For this review, take the finished solid that the model builds, in its own axes (mm). A direction names the side the tool comes from. Round coordinates to 2 decimals unless told otherwise and drop trailing zeros. Write each loop counter-clockwise with the first axis right and the second up, starting at its lowest first coordinate (ties: lowest second). Pieces come first, ordered by that corner, then holes. Notation, with made-up numbers: M 78.25,42.25 L 93.25,42.25 A20 cw 93.25,73.25 Z; hole C 4.5,-3.75 d11. An arc over 180 degrees is marked long. Answer in a Markdown table with one row per item.
```python
from build123d import *

# Parameters (mm, degrees)
F1_DEPTH = 5
F3_D     = 3.2
F3_DEPTH = 14.25
F3_TIP   = 0.9613769904
F4_R     = 5
F5_R     = 2


with BuildPart() as f1:
    # F0 (on Top) → F1 (new body)
    with BuildSketch(Plane.XY):
        Polygon((-36.25, 16.35), (-36.25, -16.35), (-26.25, -16.35), (-26.25, 1.65), (26.25, 1.65), (26.25, -16.35), (36.25, -16.35), (36.25, 16.35), align=None)
    extrude(amount=F1_DEPTH)

    # F3
    with Locations(Plane.XY.offset(5)):
        with Locations((-30, 7.35), (30, 7.35)):
            Hole(F3_D / 2, depth=F3_DEPTH)
            with Locations((0, 0, -(F3_DEPTH + F3_TIP / 2))):  # 118° drill point
                Cone(0, F3_D / 2, F3_TIP, mode=Mode.SUBTRACT)

    # F4
    f4_edges = [f1.edges().sort_by_distance(p)[0] for p in [
        (-36.25, -16.35, 2.5),
        (36.25, -16.35, 2.5),
    ]]
    fillet(f4_edges, radius=F4_R)

    # F5
    f5_edges = [f1.edges().sort_by_distance(p)[0] for p in [
        (36.25, 16.35, 2.5),
        (-36.25, 16.35, 2.5),
    ]]
    fillet(f5_edges, radius=F5_R)


solid = f1.part
```
Q1. For probe 1 along X at (y, z) = (7.5, 2.8); probe 2 along Y at (x, z) = (-30, 2.3); probe 3 along X at (y, z) = (1.5, 0.8), list the stretches that pass through material, from the lowest coordinate up.
Found:
| item | result |
|---|---|
| probe 1 | -36.25 to -31.59, -28.41 to 28.41, 31.59 to 36.25 |
| probe 2 | -16.35 to 5.75, 8.95 to 16.35 |
| probe 3 | -36.25 to -26.25, 26.25 to 36.25 |
Q2. Mouldability with a two-part tool opening along X and no side actions: class faces 1 (the face through (0, 1.65, 2)), 2 (the face through (26.25, -7, 2)), 3 (the face through (-29, -16.35, 2)), 4 (the face through (-34.82, -14.85, 2.54)) as +X half, -X half, draft (parallel to the pull), parting line (faces both ways), or undercut.
Found:
| item | result |
|---|---|
| face 1 | undercut |
| face 2 | undercut |
| face 3 | draft |
| face 4 | -X half |
Q3. Take a section at C-C (z = 1.2). State the section outline as (x, y) points.
Found:
| item | result |
|---|---|
| outline | M -36.25,-11.35 A5 ccw -31.25,-16.35 L -26.25,-16.35 L -26.25,1.65 L 26.25,1.65 L 26.25,-16.35 L 31.25,-16.35 A5 ccw 36.25,-11.35 L 36.25,14.35 A2 ccw 34.25,16.35 L -34.25,16.35 A2 ccw -36.25,14.35 Z; hole C -30,7.35 d3.2; hole C 30,7.35 d3.2 |
Q4. Take a section at A-A (x = -30). State the section outline as (y, z) points, then the cut area to 4 significant figures.
Found:
| item | result |
|---|---|
| outline | M -16.35,0 L 5.75,0 L 5.75,5 L -16.35,5 Z; M 8.95,0 L 16.35,0 L 16.35,5 L 8.95,5 Z |
| area | 147.5 mm² |
Q5. Insertion check: P1, Ø2.5, axis at x = -6, z = 3.5, coming from the -Y side. The pin has a flat end and moves straight along its axis. Give the tip position at first contact, or say it passes through.
Found:
| item | result |
|---|---|
| P1 | y = 1.65 |
Q6. Machinability: for faces 5 (the face through (-1, 7, 5)), 6 (the face through (-26.25, -7, 2)), which of the approach directions +Z, -Z, +X, -X, +Y, -Y give a long, thin tool a straight path to every point of the face, cutting with its end or side? Answer none if there is none.
Found:
| item | result |
|---|---|
| face 5 | +Z, +X, -X, +Y, -Y |
| face 6 | +Z, -Z, -Y |
Q7. Take a section at B-B (y = 0.5). State the section outline as (x, z) points.
Found:
| item | result |
|---|---|
| outline | M -36.25,0 L -26.25,0 L -26.25,5 L -36.25,5 Z; M 26.25,0 L 36.25,0 L 36.25,5 L 26.25,5 Z |
Q8. Take a section at D-D (y = 7.35). State the section outline as (x, z) points, then the cut area to 4 significant figures.
Found:
| item | result |
|---|---|
| outline | M -36.25,0 L -31.6,0 L -31.6,5 L -36.25,5 Z; M -28.4,0 L 28.4,0 L 28.4,5 L -28.4,5 Z; M 31.6,0 L 36.25,0 L 36.25,5 L 31.6,5 Z |
| area | 330.5 mm² |
